For this review, take the finished solid that the model builds, in its own axes (mm). A direction names the side the tool comes from. Coordinates: 2 decimals unless noted, no trailing zeros. Write each loop counter-clockwise with the first axis right and the second up, starting at its lowest first coordinate (ties: lowest second). Pieces come first, ordered by that corner, then holes. Notation, with made-up numbers: M 10.25,8.5 L 67.25,8.5 A18 ccw 67.25,33.5 Z; hole C 0,34.5 d5. An arc over 180 degrees is marked long. Return JSON: item names as keys, results as strings.
```python
from build123d import *

# Parameters (mm, degrees)
SKETCH1_R           = 1.5
BOSS_EXTRUDE1_DEPTH = 3
SKETCH2_W           = 22.5
SKETCH2_H           = 6
BOSS_EXTRUDE2_DEPTH = 20
SKETCH3_W           = 18.5
SKETCH3_H           = 19
CUT_EXTRUDE1_DEPTH  = 10
SKETCH4_W           = 3.85
SKETCH4_H           = 6
BOSS_EXTRUDE3_DEPTH = 2
SKETCH5_R           = 1.5
CUT_EXTRUDE2_DEPTH  = 2
SKETCH6_W           = 6
SKETCH6_H           = 2
BOSS_EXTRUDE4_DEPTH = 2
SKETCH7_W           = 2
SKETCH7_H           = 6
BOSS_EXTRUDE5_DEPTH = 28
SKETCH8_W           = 6
SKETCH8_H           = 2
BOSS_EXTRUDE6_DEPTH = 2
SKETCH9_W           = 2
SKETCH9_H           = 6
BOSS_EXTRUDE7_DEPTH = 28
SKETCH11_W          = 6
SKETCH11_H          = 4
BOSS_EXTRUDE8_DEPTH = 31


with BuildPart() as part:
    # Sketch1 → Boss-Extrude1 (new body)
    with BuildSketch(Plane(origin=(0, 0, 0), x_dir=(1, 0, 0), z_dir=(0, 1, 0))):
        with BuildLine():
            Line((2.645751311, 3), (25.854248689, 3))
            ThreePointArc((25.854248689, 3), (32.5, 0), (25.854248689, -3))
            Line((25.854248689, -3), (2.645751311, -3))
            ThreePointArc((2.645751311, -3), (-4, 0), (2.645751311, 3))
        make_face()
        Circle(SKETCH1_R, mode=Mode.SUBTRACT)
        with Locations((28.5, 0)):
            Circle(SKETCH1_R, mode=Mode.SUBTRACT)
    extrude(amount=BOSS_EXTRUDE1_DEPTH)

    # Sketch2 → Boss-Extrude2 (add)
    with BuildSketch(Plane(origin=(0, 3, 0), x_dir=(1, 0, 0), z_dir=(0, 1, 0))):
        with Locations((14.25, 0)):
            Rectangle(SKETCH2_W, SKETCH2_H)
    extrude(amount=BOSS_EXTRUDE2_DEPTH)

    # Sketch3 → Cut-Extrude1 (cut)
    with BuildSketch(Plane.XY.offset(3)):
        with Locations((14.25, 11.5)):
            Rectangle(SKETCH3_W, SKETCH3_H)
    extrude(amount=-CUT_EXTRUDE1_DEPTH, mode=Mode.SUBTRACT)

    # Sketch4 → Boss-Extrude3 (add)
    with BuildSketch(Plane(origin=(0, 23, 0), x_dir=(1, 0, 0), z_dir=(0, 1, 0))):
        with BuildLine():
            Line((11.604248689, 3), (16.895751311, 3))
            ThreePointArc((16.895751311, 3), (14.25, 4), (11.604248689, 3))
        make_face()
        with Locations((27.425, 0)):
            Rectangle(SKETCH4_W, SKETCH4_H)
        with Locations((1.075, 0)):
            Rectangle(SKETCH4_W, SKETCH4_H)
        with BuildLine():
            ThreePointArc((11.604248689, -3), (14.25, -4), (16.895751311, -3))
            Line((16.895751311, -3), (11.604248689, -3))
        make_face()
    extrude(amount=-BOSS_EXTRUDE3_DEPTH)

    # Sketch5 → Cut-Extrude2 (cut)
    with BuildSketch(Plane(origin=(0, 23, 0), x_dir=(1, 0, 0), z_dir=(0, 1, 0))):
        with Locations((14.25, 0)):
            Circle(SKETCH5_R)
    extrude(amount=-CUT_EXTRUDE2_DEPTH, mode=Mode.SUBTRACT)

    # Sketch6 → Boss-Extrude4 (add)
    with BuildSketch(Plane.ZY.offset(0.85)):
        with Locations((0, 22)):
            Rectangle(SKETCH6_W, SKETCH6_H)
    extrude(amount=BOSS_EXTRUDE4_DEPTH)

    # Sketch7 → Boss-Extrude5 (add)
    with BuildSketch(Plane(origin=(0, 23, 0), x_dir=(1, 0, 0), z_dir=(0, 1, 0))):
        with Locations((-1.85, 0)):
            Rectangle(SKETCH7_W, SKETCH7_H)
    extrude(amount=BOSS_EXTRUDE5_DEPTH)

    # Sketch8 → Boss-Extrude6 (add)
    with BuildSketch(Plane(origin=(29.35, 0, 0), x_dir=(0, 0, -1), z_dir=(1, 0, 0))):
        with Locations((0, 22)):
            Rectangle(SKETCH8_W, SKETCH8_H)
    extrude(amount=BOSS_EXTRUDE6_DEPTH)

    # Sketch9 → Boss-Extrude7 (add)
    with BuildSketch(Plane(origin=(0, 23, 0), x_dir=(1, 0, 0), z_dir=(0, 1, 0))):
        with Locations((30.35, 0)):
            Rectangle(SKETCH9_W, SKETCH9_H)
    extrude(amount=BOSS_EXTRUDE7_DEPTH)

    # Sketch11 → Boss-Extrude8 (add)
    with BuildSketch(Plane.ZY.offset(-29.35)):
        with Locations((0, 49)):
            Rectangle(SKETCH11_W, SKETCH11_H)
    extrude(amount=BOSS_EXTRUDE8_DEPTH)


solid = part.part
```
1. Clearance check with flat-ended pins moving along their axes: pin 1 Ø2.5 at (x, z) = (12, -1) entering from -Y; pin 2 Ø3 at (y, z) = (34, -0.5) entering from -X; pin 3 Ø4 at (y, z) = (16.5, -2) entering from +X; pin 4 Ø1.5 at (y, z) = (5, 0) entering from -X. State where each tip first meets the part, or that it passes through.
Checks:
{"pin 1": "y = 0", "pin 2": "x = -2.85", "pin 3": "x = 25.5", "pin 4": "x = 3"}
2. Draft analysis for pull direction X (two halves, no side actions). For faces 1 (the face through (32.5, 1.5, -0.1)), 2 (the face through (25.5, 12, 0)), 3 (the face through (15, 0, 0)), state which applies: +X half, -X half, draft (parallel to the pull), parting line (faces both ways), or undercut.
Checks:
{"face 1": "undercut", "face 2": "+X half", "face 3": "draft"}
3. We need section B-B (x = 14.25). State the section outline as (y, z) points, plus the area to 3 significant figures.
Checks:
{"outline": "M 0,-3 L 2,-3 L 2,3 L 0,3 Z; M 21,-4 L 23,-4 L 23,-1.5 L 21,-1.5 Z; M 21,1.5 L 23,1.5 L 23,4 L 21,4 Z; M 47,-3 L 51,-3 L 51,3 L 47,3 Z", "area": "46.0 mm2"}
4. We need section C-C (y = 11). State the section outline as (x, z) points.
Checks:
{"outline": "M 3,-3 L 5,-3 L 5,3 L 3,3 Z; M 23.5,-3 L 25.5,-3 L 25.5,3 L 23.5,3 Z"}
5. We need section A-A (z = 0). Give the number of separate pieces and of enclosed holes in the cut face, plus the area to 3 significant figures.
Checks:
{"separate pieces": "3", "enclosed holes": "1", "area": "440 mm2"}
6. Wall thickness on L1, parallel to Y at x = 1, z = -2.75; L2, parallel to X at y = 0.8, z = 0; L3, parallel to Y at x = 17.5, z = -0.25: over which ranges is each line inside the solid? List them lowest first. Write a range as from..to.
Checks:
{"L1": "0..3, 21..23, 47..51", "L2": "-4..-1.5, 1.5..27, 30..32.5", "L3": "0..2, 21..23, 47..51"}
7. For faces 4 (the face through (14, 23, 2)), 5 (the face through (12.75, 22.01, -0.07)), 6 (the face through (-2.85, 36, 0)), 7 (the face through (0, 3, 2)), list the 3-axis set-ups (+Z, -Z, +X, -X, +Y, -Y) from which the entire face can be reached by the end or side of a thin tool; tool diameter is ignored.
Checks:
{"face 4": "+Z, -Z", "face 5": "none", "face 6": "+Z, -Z, -X, +Y", "face 7": "+Z, -Z, -X"}
8. We need section D-D (x = 22.5). State the section outline as (y, z) points.
Checks:
{"outline": "M 0,-3 L 2,-3 L 2,3 L 0,3 Z; M 21,-3 L 23,-3 L 23,3 L 21,3 Z; M 47,-3 L 51,-3 L 51,3 L 47,3 Z"}
